The drawing under review shows one solid part. Ordinate dimensions are in mm from its lowest x, y, z. Give positions to 0.01 mm unless a question says otherwise; leave off trailing zeros. Write each loop counter-clockwise with the first axis right and the second up, starting at its lowest first coordinate (ties: lowest second). Pieces come first, ordered by that corner, then holes. Notation, with made-up numbers: (-35, 84) -> (-12, 84) arc R25 cw to (-12, 114) -> close; hole circle Ø1 at (62.5, 50). An arc over 180 degrees is marked (long way). Put each result on its own line as item: value. Start each with the question number.
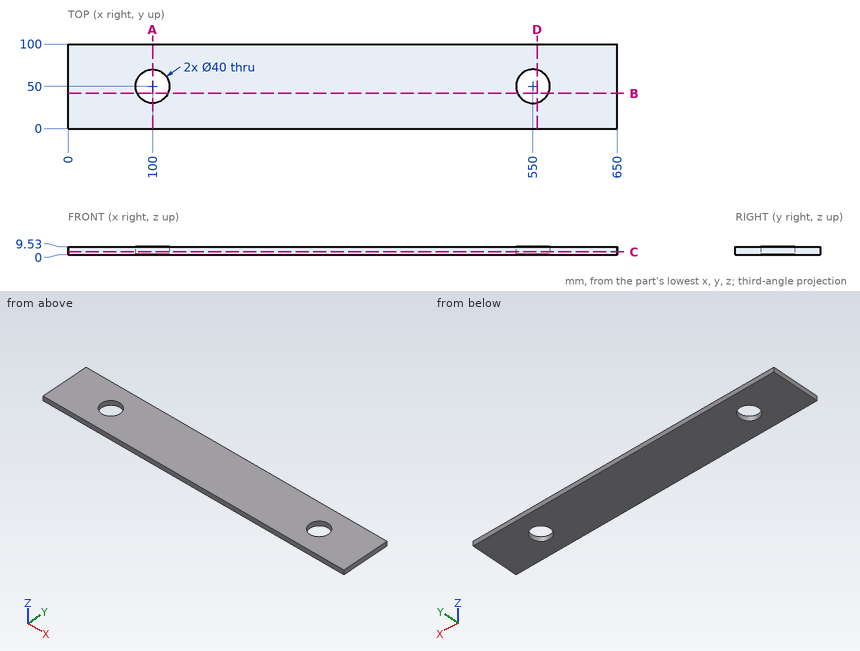
Q1. Take a section at C-C on z = 3.25. Give the boundary of the cut face in (x, y).
Q2. To check wall thickness, follow probe 1 along X at (y, z) = (63, 2); probe 2 along X at (y, z) = (65, 3); probe 3 along Y at (x, z) = (550, 2). State the ranges of each line that lie inside material, in increasing order. Write a range as from..to.
Q3. Take a section at B-B on y = 41.5. Give the boundary of the cut face in (x, z).
Q4. For pin 1 (5 mm diameter, centred on y = 80.5, z = 4.5, fed in from -X), flat-tipped, find the tip position at first contact; note if it passes through.
Q5. Take a section at A-A on x = 100. Give the boundary of the cut face in (y, z).
Q6. Take a section at D-D on x = 555. Give the boundary of the cut face in (y, z).
Result:
1. outline: (0, 0) -> (650, 0) -> (650, 100) -> (0, 100) -> close; hole circle Ø40 at (100, 50); hole circle Ø40 at (550, 50)
2. probe 1: x = 0..84.8, 115.2..534.8, 565.2..650
2. probe 2: x = 0..86.77, 113.23..536.77, 563.23..650
2. probe 3: y = 0..30, 70..100
3. outline: (0, 0) -> (81.9, 0) -> (81.9, 9.53) -> (0, 9.53) -> close; (118.1, 0) -> (531.9, 0) -> (531.9, 9.53) -> (118.1, 9.53) -> close; (568.1, 0) -> (650, 0) -> (650, 9.53) -> (568.1, 9.53) -> close
4. pin 1: stops at x = 0
5. outline: (0, 0) -> (30, 0) -> (30, 9.53) -> (0, 9.53) -> close; (70, 0) -> (100, 0) -> (100, 9.53) -> (70, 9.53) -> close
6. outline: (0, 0) -> (30.64, 0) -> (30.64, 9.53) -> (0, 9.53) -> close; (69.36, 0) -> (100, 0) -> (100, 9.53) -> (69.36, 9.53) -> close
